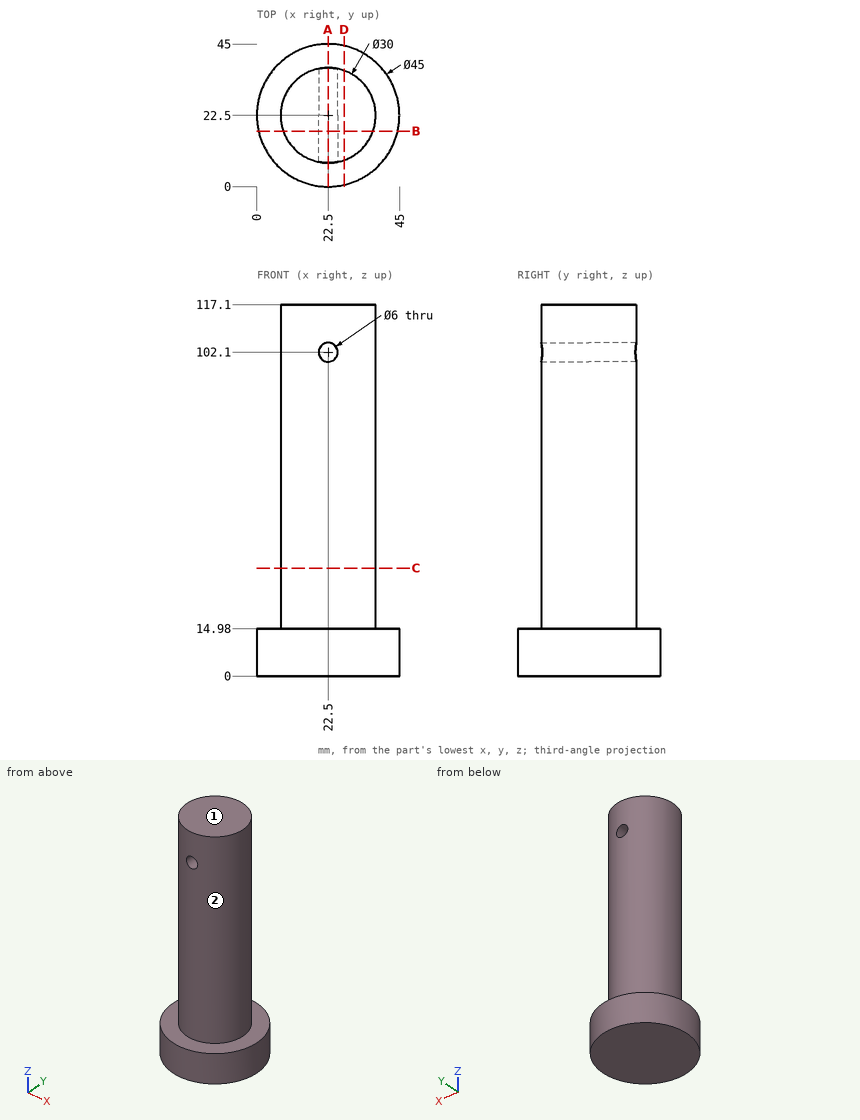
The drawing under review shows one solid part. Ordinate dimensions are in mm from its lowest x, y, z. A direction names the side the tool comes from. Round coordinates to 2 decimals unless told otherwise and drop trailing zeros. Loops run counter-clockwise (first coordinate to the right, second up) from the corner with the lowest first, then second, coordinate; pieces in that order, holes last.
Item 1: Take a section at D-D (x = 27.5). Write out the cut boundary in (y, z), then the cut area to 3 significant figures.
Determined:
outline: (0.56, 0) - (44.44, 0) - (44.44, 14.98) - (36.64, 14.98) - (36.64, 117.1) - (8.36, 117.1) - (8.36, 14.98) - (0.56, 14.98) - close
area: 3,550 mm2
Item 2: For the marked faces 1 and 2, list the 3-axis set-ups (+Z, -Z, +X, -X, +Y, -Y) from which the entire face can be reached by the end or side of a thin tool; tool diameter is ignored.
Determined:
face 1: +Z, +X, -X, +Y, -Y
face 2: +Z
Item 3: For line 1 (Z direction, x = 22.5, y = 27.75); line 2 (X direction, y = 19.25, z = 102.1); line 3 (Z direction, x = 42, y = 32), list the stretches that pass through material, from the lowest coordinate up.
Determined:
line 1: z = 0 to 99.1, 105.1 to 117.1
line 2: x = 7.86 to 19.5, 25.5 to 37.14
line 3: z = 0 to 14.98
Item 4: Take a section at A-A (x = 22.5). Write out the cut boundary in (y, z).
Determined:
outline: (0, 0) - (45, 0) - (45, 14.98) - (37.5, 14.98) - (37.5, 99.1) - (7.5, 99.1) - (7.5, 14.98) - (0, 14.98) - close; (7.5, 105.1) - (37.5, 105.1) - (37.5, 117.1) - (7.5, 117.1) - close
Item 5: Take a section at C-C (z = 34). Write out the cut boundary in (x, y).
Determined:
outline: circle Ø30 at (22.5, 22.5)
Item 6: Clearance check with flat-ended pins moving along their axes: pin 1 Ø3.5 at (x, z) = (22.5, 102.1) entering from -Y; pin 2 Ø12 at (y, z) = (13, 83) entering from +X; pin 3 Ø1.5 at (y, z) = (20.5, 35) entering from +X; pin 4 Ø4 at (x, z) = (29, 16.5) entering from -Y. State where each tip first meets the part, or that it passes through.
Determined:
pin 1: passes through
pin 2: stops at x = 37.09
pin 3: stops at x = 37.45
pin 4: stops at y = 0.61
Item 7: Take a section at B-B (y = 17.5). Write out the cut boundary in (x, z), then the cut area to 3 significant figures.
Determined:
outline: (0.56, 0) - (44.44, 0) - (44.44, 14.98) - (36.64, 14.98) - (36.64, 117.1) - (8.36, 117.1) - (8.36, 14.98) - (0.56, 14.98) - close; hole circle Ø6 at (22.5, 102.1)
area: 3,520 mm2
